```python
from build123d import *

# Parameters (mm, degrees)
SKETCH_1_W          = 200
SKETCH_1_H          = 100
EXTRUDE_1_DEPTH     = 15
EXTRUDE_2_DEPTH     = 20
CUT_EXTRUDE_2_DEPTH = 201
SKETCH_4_R          = 7.5
CUT_EXTRUDE_3_DEPTH = 101
FILLET_2_R          = 10


with BuildPart() as part:
    # 스케치1 → 보스-돌출1 (new body)
    with BuildSketch(Plane(origin=(0, 0, 0), x_dir=(1, 0, 0), z_dir=(0, 1, 0))):
        with Locations((100, 50)):
            Rectangle(SKETCH_1_W, SKETCH_1_H)
    extrude(amount=EXTRUDE_1_DEPTH)

    # 스케치2 → 보스-돌출2 (add)
    with BuildSketch(Plane.XY):
        with BuildLine():
            Line((50, 0), (120, 0))
            Line((120, 0), (120, 80))
            ThreePointArc((120, 80), (85, 115), (50, 80))
            Line((50, 80), (50, 0))
        make_face()
    extrude(amount=-EXTRUDE_2_DEPTH)

    # 스케치3 → 컷-돌출2 (cut, through all)
    with BuildSketch(Plane(origin=(200, 0, 0), x_dir=(0, 0, -1), z_dir=(1, 0, 0))):
        Polygon((25, 0), (25, 5), (35, 5), (35, 10), (45, 10), (45, 5), (55, 5), (55, 10), (65, 10), (65, 5), (75, 5), (75, 0), align=None)
    extrude(amount=-CUT_EXTRUDE_2_DEPTH, mode=Mode.SUBTRACT)

    # 스케치4 → 컷-돌출3 (cut, through all)
    with BuildSketch(Plane.XY):
        with Locations((85, 80)):
            Circle(SKETCH_4_R)
    extrude(amount=-CUT_EXTRUDE_3_DEPTH, mode=Mode.SUBTRACT)

    # 필렛2
    fillet_2_edges = [part.edges().sort_by_distance(p)[0] for p in [
        (50, 15, -10),
        (120, 15, -10),
    ]]
    fillet(fillet_2_edges, radius=FILLET_2_R)


solid = part.part
```
Verification items for the finished model (mm, model axes). A direction names the side the tool comes from. Coordinates: 2 decimals unless noted, no trailing zeros. Write each loop counter-clockwise with the first axis right and the second up, starting at its lowest first coordinate (ties: lowest second). Pieces come first, ordered by that corner, then holes. Notation, with made-up numbers: (-40, 32.5) - (-24, 32.5) arc R24 ccw to (-24, 42.5) - close; hole circle Ø3 at (54.5, -40). An arc over 180 degrees is marked (long way). Write item = value, one per line.
Q1. Cross-section at C-C (y = 35). Enter the section's corners in (x, z).
Answer:
outline = (50, -20) - (120, -20) - (120, 0) - (50, 0) - close
Q2. Go/stop test with flat-tipped pins: pin 1 Ø12 at (x, z) = (89, -53) entering from +Y; pin 2 Ø5 at (x, z) = (52, -49) entering from -Y; pin 3 Ø6 at (y, z) = (61, -8.5) entering from -X; pin 4 Ø5.5 at (x, y) = (76, 6.5) entering from +Z. Record where each tip stops, or that it passes through.
Answer:
pin_1 = 15
pin_2 = 5
pin_3 = 50
pin_4 = 0
Q3. Access from +Z, -Z, +X, -X, +Y, -Y to the whole of each face (thin tool, end or side, straight path). Record for faces 1 (the face through (50, 53, -10)), 2 (the face through (101, 7, -55)), 3 (the face through (85.77, 114.99, -9.86)), 4 (the face through (84, 66, -20)).
Answer:
face_1 = +Z, -Z, -X, +Y
face_2 = +X, -X, -Y
face_3 = +Z, -Z, +Y
face_4 = -Z, +X, -X, +Y
Q4. Cross-section at D-D (z = -61). Enter the section's corners in (x, y), plus the area to 3 significant figures.
Answer:
outline = (0, 10) - (200, 10) - (200, 15) - (0, 15) - close
area = 1,000 mm²
Q5. Material ranges on L1, parallel to Z at x = 168.5, y = 7; L2, parallel to Y at x = 85, z = -12; L3, parallel to Y at x = 138.5, z = -94, recorded low to high. Write a range as from..to.
Answer:
L1 = -100..-65, -55..-45, -35..0
L2 = 0..72.5, 87.5..115
L3 = 0..15
Q6. Cross-section at A-A (x = 85). Enter the section's corners in (y, z), plus the area to 3 significant figures.
Answer:
outline = (0, -100) - (15, -100) - (15, -20) - (72.5, -20) - (72.5, 0) - (0, 0) - (0, -25) - (5, -25) - (5, -35) - (10, -35) - (10, -45) - (5, -45) - (5, -55) - (10, -55) - (10, -65) - (5, -65) - (5, -75) - (0, -75) - close; (87.5, -20) - (115, -20) - (115, 0) - (87.5, 0) - close
area = 2,850 mm²
Q7. Mould release check, pull along Z, two halves, no side actions. Record for faces 5 (the face through (99, 0, -12)), 6 (the face through (101, 2, -25)), 7 (the face through (101, 5, -50)), 8 (the face through (76, 44, 0)): released by +Z, released by -Z, zero draft, split by the parting line, or undercut.
Answer:
face_5 = zero draft
face_6 = undercut
face_7 = undercut
face_8 = released by +Z
Q8. Cross-section at B-B (x = 160). Enter the section's corners in (y, z), plus the area to 3 significant figures.
Answer:
outline = (0, -100) - (15, -100) - (15, 0) - (0, 0) - (0, -25) - (5, -25) - (5, -35) - (10, -35) - (10, -45) - (5, -45) - (5, -55) - (10, -55) - (10, -65) - (5, -65) - (5, -75) - (0, -75) - close
area = 1,150 mm²
